```python
from build123d import *

# Parameters (mm, degrees)
SKETCH1_W           = 70
SKETCH1_H           = 115
SKETCH1_R           = 4.5
SKETCH1_R_2         = 1.75
BOSS_EXTRUDE1_DEPTH = 1


with BuildPart() as part:
    # Sketch1 → Boss-Extrude1 (new body)
    with BuildSketch(Plane(origin=(0, 0, 0), x_dir=(0, 0, -1), z_dir=(1, 0, 0))):
        Rectangle(SKETCH1_W, SKETCH1_H)
        Circle(SKETCH1_R, mode=Mode.SUBTRACT)
        with Locations((0, 8)):
            Circle(SKETCH1_R_2, mode=Mode.SUBTRACT)
        with Locations((8, 0)):
            Circle(SKETCH1_R_2, mode=Mode.SUBTRACT)
        with Locations((0, -8)):
            Circle(SKETCH1_R_2, mode=Mode.SUBTRACT)
        with Locations((-8, 0)):
            Circle(SKETCH1_R_2, mode=Mode.SUBTRACT)
        with Locations((-6, 37.5)):
            Circle(SKETCH1_R_2, mode=Mode.SUBTRACT)
        with Locations(Location((6, 37.5, 0), (0, 0, 180))):
            Circle(SKETCH1_R_2, mode=Mode.SUBTRACT)
        with Locations((6, -37.5)):
            Circle(SKETCH1_R_2, mode=Mode.SUBTRACT)
        with Locations(Location((-6, -37.5, 0), (0, 0, 180))):
            Circle(SKETCH1_R_2, mode=Mode.SUBTRACT)
    extrude(amount=BOSS_EXTRUDE1_DEPTH)


solid = part.part
```
Design review of the part built by this model. Coordinates are the model's own, in mm. Coordinates: 2 decimals unless noted, no trailing zeros. Order: outer loops, then holes, each group sorted by start corner. A loop starts at its lowest first (then second) coordinate and runs counter-clockwise, first axis right, second up.
1) Clearance check with a flat-ended pin moving along its axis: pin 1 (2 mm diameter, centred on y = 0, z = 8, fed in from +X). State where the tip first meets the part, or that it passes through.
2) Mouldability with a two-part tool opening along Y and no side actions: class faces 1 (the flat face through (1, 14, 0)), 2 (the cylindrical face through (0.49, -39.21, -5.62)) as +Y half, -Y half, draft (parallel to the pull), parting line (faces both ways), or undercut.
3) Take a section at B-B, the plane x = 0.2. State how many separate pieces and enclosed holes the cut face has, and give its area (3 significant figures).
4) Wall thickness on line 1 along Y through (x, z) = (0.45, 0); line 2 along Y through (x, z) = (0.7, -8): over which ranges is each line inside the solid? List them lowest first.
5) Take a section at A-A, the plane y = -37.5. Give the boundary of the cut face in (x, z), and give its area (3 significant figures).
6) Take a section at D-D, the plane y = -8. Give the boundary of the cut face in (x, z).
7) Take a section at C-C, the plane z = 0. Give the boundary of the cut face in (x, y), and give its area (3 significant figures).
Returned:
1. pin 1: passes through
2. face 1: draft
2. face 2: undercut
3. separate pieces: 1
3. enclosed holes: 9
3. area: 7,910 mm2
4. line 1: y = -57.5 to -9.75, -6.25 to -4.5, 4.5 to 6.25, 9.75 to 57.5
4. line 2: y = -57.5 to -1.75, 1.75 to 57.5
5. outline: (0, -35) - (1, -35) - (1, -7.75) - (0, -7.75) - close; (0, -4.25) - (1, -4.25) - (1, 4.25) - (0, 4.25) - close; (0, 7.75) - (1, 7.75) - (1, 35) - (0, 35) - close
5. area: 63.0 mm2
6. outline: (0, -35) - (1, -35) - (1, -1.75) - (0, -1.75) - close; (0, 1.75) - (1, 1.75) - (1, 35) - (0, 35) - close
7. outline: (0, -57.5) - (1, -57.5) - (1, -9.75) - (0, -9.75) - close; (0, -6.25) - (1, -6.25) - (1, -4.5) - (0, -4.5) - close; (0, 4.5) - (1, 4.5) - (1, 6.25) - (0, 6.25) - close; (0, 9.75) - (1, 9.75) - (1, 57.5) - (0, 57.5) - close
7. area: 99.0 mm2
